The model under review builds one solid part; all positions refer to its coordinate system, in mm. A direction names the side the tool comes from. Round coordinates to 2 decimals unless told otherwise and drop trailing zeros. Write each loop counter-clockwise with the first axis right and the second up, starting at its lowest first coordinate (ties: lowest second). Pieces come first, ordered by that corner, then holes. Notation, with made-up numbers: M 76.5,9 L 117.5,9 A10 ccw 117.5,16 Z; hole C 24,25.25 d8. An arc over 180 degrees is marked long. One line per item, written item: value. Start each with the question number.
1) Take a section at A-A, the plane x = 22.5. Write out the cut boundary in (y, z) (3 decimals), and give its area (3 significant figures).
2) Wall thickness on probe 1 along Y at (x, z) = (-9.5, 1.4); probe 2 along Y at (x, z) = (16, 1.2); probe 3 along X at (y, z) = (-2, 0.2): over which ranges is each line inside the solid? List them lowest first.
3) For P1, Ø2.5, axis at x = 13, y = 1, coming from the -Z side; P2, Ø2, axis at x = -1, y = 3, coming from the -Z side, all flat-tipped, find the tip position at first contact; note any pin that passes through.
4) Tool access review of faces 1 (the face through (5, 2.899, 1)), 2 (the face through (5.4, 3.1, 0)): name each direction out of +Z, -Z, +X, -X, +Y, -Y from which nothing blocks a thin tool from reaching the whole face with its end or side.
5) Mouldability with a two-part tool opening along X and no side actions: class faces 3 (the face through (-26.057, 0, 2)), 4 (the face through (13, 0, 0.32)), 5 (the face through (5, 0, 3.175)) as +X half, -X half, draft (parallel to the pull), parting line (faces both ways), or undercut.
from build123d import *

# Parameters (mm, degrees)
F0_W     = 63.881
F0_H     = 8.128
F1_DEPTH = 3.175
F2_T     = -1.524
F3_R     = 1.2319
F4_DEPTH = 1.33086


with BuildPart() as f1:
    # F0 (on Top) → F1 (new body)
    with BuildSketch(Plane.XY):
        with Locations((5.883156, 0.358789)):
            Rectangle(F0_W, F0_H)
    extrude(amount=F1_DEPTH)

    # F2
    f2_openings = [f1.faces().sort_by_distance(p)[0] for p in [
        (5.883156, 0.358789, 0),
    ]]
    offset(amount=F2_T, openings=f2_openings)

    # F3 (on face) → F4 (join)
    with BuildSketch(Plane(origin=(0, 0, 1.651), x_dir=(1, 0, 0), z_dir=(0, 0, -1))):
        with Locations((28.349456, -0.358789)):
            Circle(F3_R)
        with Locations((20.729456, -0.358789)):
            Circle(F3_R)
        with Locations((13.109456, -0.358789)):
            Circle(F3_R)
        with Locations((5.489456, -0.358789)):
            Circle(F3_R)
        with Locations((-2.130544, -0.358789)):
            Circle(F3_R)
        with Locations((-9.750544, -0.358789)):
            Circle(F3_R)
        with BuildLine():
            ThreePointArc((-18.602444, -0.358789), (-17.370544, -1.590689), (-16.138644, -0.358789))
            ThreePointArc((-16.138644, -0.358789), (-17.370544, 0.873111), (-18.602444, -0.358789))
        make_face()
    extrude(amount=F4_DEPTH)


solid = f1.part
Checked values:
1. outline: M -3.705,0 L -2.181,0 L -2.181,1.651 L 2.899,1.651 L 2.899,0 L 4.423,0 L 4.423,3.175 L -3.705,3.175 Z
1. area: 17.4 mm2
2. probe 1: y = -3.71 to -2.18, -0.85 to 1.56, 2.9 to 4.42
2. probe 2: y = -3.71 to -2.18, 2.9 to 4.42
2. probe 3: x = -26.06 to -24.53, 36.3 to 37.82
3. P1: stops at z = 0.32
3. P2: stops at z = 0
4. face 1: -Z
4. face 2: -Z, +X, -X, +Y, -Y
5. face 3: -X half
5. face 4: undercut
5. face 5: draft
